Can you work these out from the drawing? Everything is in mm from the part's minimum corner. Give positions to 0.01 mm unless a question says otherwise; leave off trailing zeros. Write each loop counter-clockwise with the first axis right and the second up, starting at its lowest first coordinate (ties: lowest second). Pieces come first, ordered by that corner, then holes. Notation, with made-up numbers: (10.25, 30.25) -> (37.25, 30.25) arc R9 ccw to (37.25, 40.25) -> close; hole circle Ø6 at (15, 3). An arc over 180 degrees is marked (long way). Write item = value, one per line. Start each with the question number.
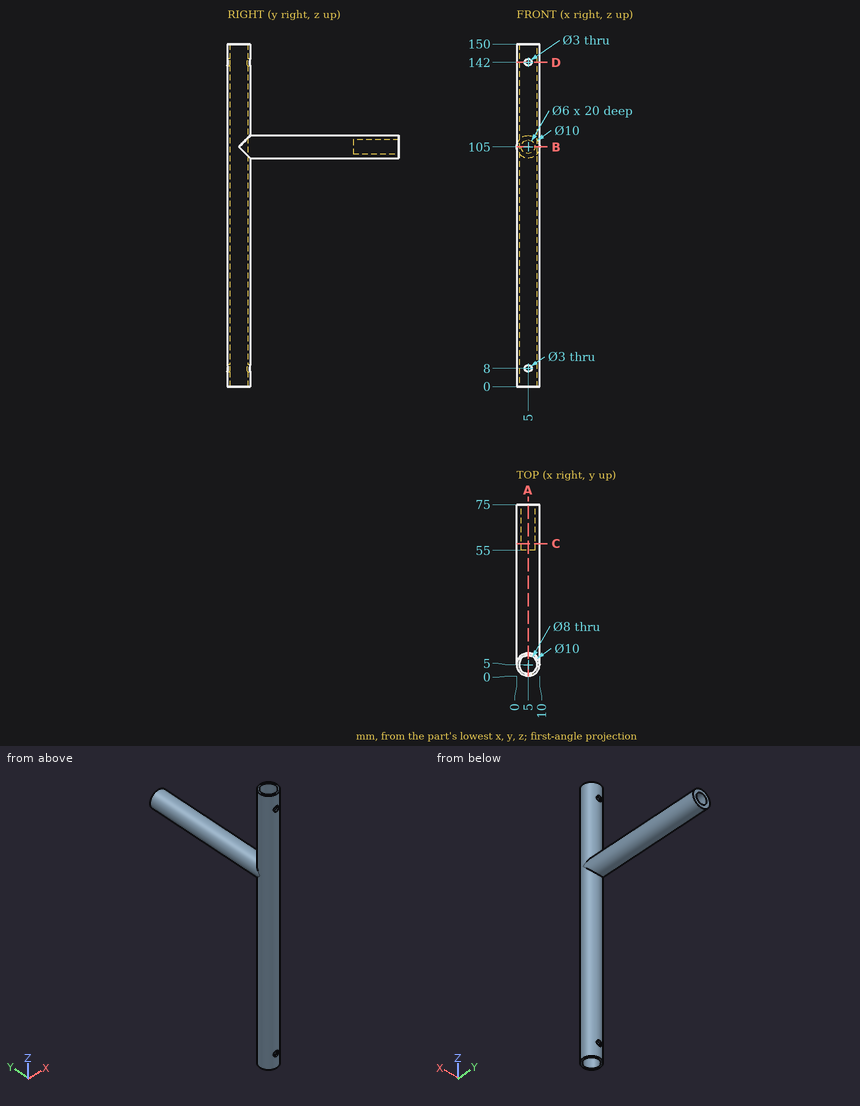
(1) I'm going to push flat-ended pins straight in: pin 1 (5 mm diameter, centred on x = 5, z = 142, fed in from +Y); pin 2 (5 mm diameter, centred on x = 4, z = 121, fed in from -Y); pin 3 (1.5 mm diameter, centred on x = 2.5, z = 25.5, fed in from -Y); pin 4 (2 mm diameter, centred on x = 7.5, z = 23.5, fed in from +Y). Where does each tip first touch, or does it pass through?
(2) Imagine slicing it at B-B (z = 105). Please give me the cut outline in (x, y).
(3) Imagine slicing it at C-C (y = 58). Please give me the cut outline in (x, z).
(4) If I drill on line 1 along Y through (x, z) = (4.75, 68); line 2 along X through (y, z) = (9, 8); line 3 along Y through (x, z) = (6, 125), over which ranges is the centre line in solid material (lowest first)? Write a range as from..to.
(5) Imagine slicing it at A-A (x = 5). State how many separate pieces and enclosed holes the cut face has, then the cut area to 3 significant figures.
(6) Imagine slicing it at D-D (z = 142). Please give me the cut outline in (x, y), then the cut area to 3 significant figures.
Answers below:
q1.pin_1 = 10
q1.pin_2 = 0
q1.pin_3 = 0.32
q1.pin_4 = 9.77
q2.outline = (0, 5) arc R5 ccw to (10, 5) -> (10, 75) -> (8, 75) -> (8, 55) -> (2, 55) -> (2, 75) -> (0, 75) -> close; hole circle Ø8 at (5, 5)
q3.outline = circle Ø10 at (5, 105); hole circle Ø6 at (5, 105)
q4.line_1 = 0.01..1.01, 8.99..9.99
q4.line_2 = 2..3.5, 6.5..8
q4.line_3 = 0.1..1.13, 8.87..9.9
q5.separate_pieces = 6
q5.enclosed_holes = 0
q5.area = 818 mm^2
q6.outline = (3.5, 0.23) -> (3.5, 1.29) arc R4 cw to (3.5, 8.71) -> (3.5, 9.77) arc R5 ccw to start; (6.5, 0.23) arc R5 ccw to (6.5, 9.77) -> (6.5, 8.71) arc R4 cw to (6.5, 1.29) -> close
q6.area = 22.2 mm^2
